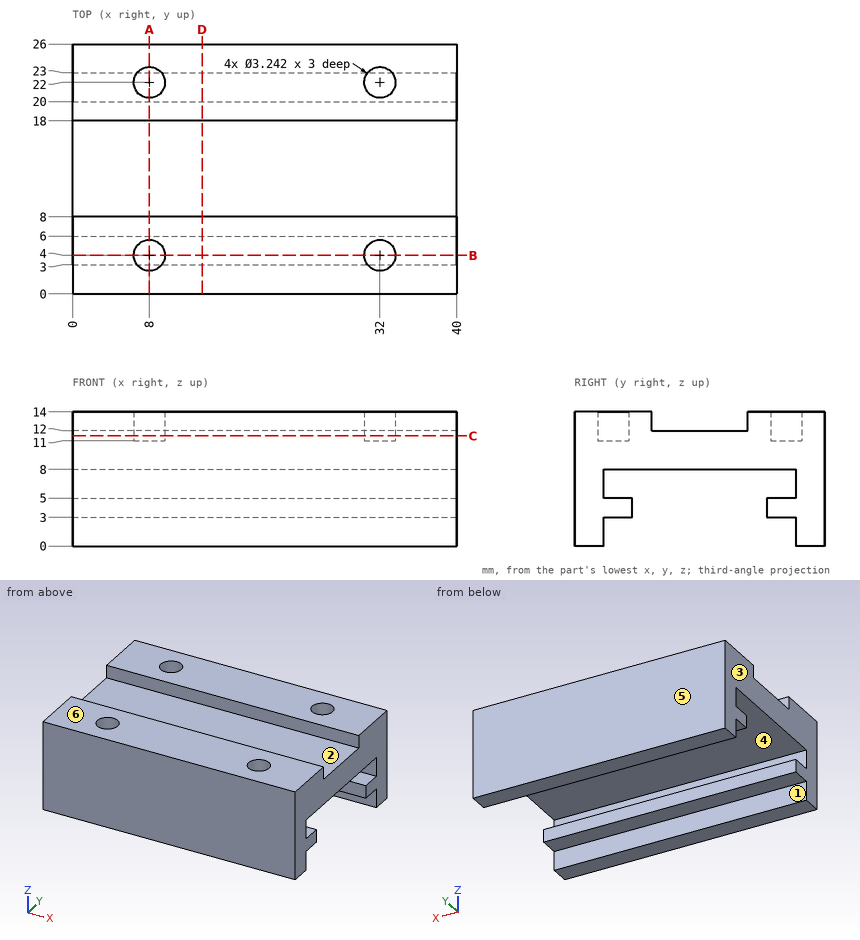
Part print with two shaded views. Sizes in mm from the minimum x, y, z corner. A direction names the side the tool comes from. Coordinates: 2 decimals unless noted, no trailing zeros. Write each loop counter-clockwise with the first axis right and the second up, starting at its lowest first coordinate (ties: lowest second). Pieces come first, ordered by that corner, then holes. Notation, with made-up numbers: (30, 26) - (62, 26) arc R19 cw to (62, 44) - close; hole circle Ø3 at (41.5, -15.75). An arc over 180 degrees is marked (long way). One line per item, written item: value. Start each with the question number.
1. Mould opens along Y. For the marked faces 4, 5 and 6 say: released by +Y, released by -Y, zero draft, split by the parting line, or undercut.
2. Tool access for the marked faces 1, 2 and 3: list every direction of +Z, -Z, +X, -X, +Y, -Y with a clear straight run to the whole face (end or side of a thin tool).
3. Slice it at B-B (y = 4). Write the cut outline in (x, z), plus the area to 3 significant figures.
4. Flat gauge pins, fed straight in: pin 1 (5 mm diameter, centred on x = 26.5, y = 13.5, fed in from +Z); pin 2 (2.5 mm diameter, centred on x = 25.5, y = 21.5, fed in from -Z); pin 3 (1 mm diameter, centred on x = 32.5, y = 4.5, fed in from +Z). Where does each tip first touch, or does it go through?
5. Slice it at C-C (z = 11.5). Write the cut outline in (x, y).
6. Slice it at A-A (x = 8). Write the cut outline in (y, z), plus the area to 3 significant figures.
7. Probe line 1 (Y direction, x = 8, z = 13.35); line 2 (X direction, y = 4, z = 12.95); line 3 (Y direction, x = 32, z = 11.8). List the from-to ranges inside material, lowest first. Write a range as from..to.
8. Slice it at D-D (x = 13.5). Write the cut outline in (y, z).
Answers below:
1. face 4: undercut
1. face 5: released by +Y
1. face 6: zero draft
2. face 1: -Z, +X, -X
2. face 2: +Z, +X, -X
2. face 3: +Z, -Z, -X, +Y, -Y
3. outline: (0, 3) - (40, 3) - (40, 5) - (0, 5) - close; (0, 8) - (40, 8) - (40, 14) - (33.62, 14) - (33.62, 11) - (30.38, 11) - (30.38, 14) - (9.62, 14) - (9.62, 11) - (6.38, 11) - (6.38, 14) - (0, 14) - close
3. area: 301 mm^2
4. pin 1: stops at z = 12
4. pin 2: stops at z = 3
4. pin 3: stops at z = 11
5. outline: (0, 0) - (40, 0) - (40, 26) - (0, 26) - close; hole circle Ø3.24 at (8, 4); hole circle Ø3.24 at (8, 22); hole circle Ø3.24 at (32, 4); hole circle Ø3.24 at (32, 22)
6. outline: (0, 0) - (3, 0) - (3, 3) - (6, 3) - (6, 5) - (3, 5) - (3, 8) - (23, 8) - (23, 5) - (20, 5) - (20, 3) - (23, 3) - (23, 0) - (26, 0) - (26, 14) - (23.62, 14) - (23.62, 11) - (20.38, 11) - (20.38, 14) - (18, 14) - (18, 12) - (8, 12) - (8, 14) - (5.62, 14) - (5.62, 11) - (2.38, 11) - (2.38, 14) - (0, 14) - close
6. area: 177 mm^2
7. line 1: y = 0..2.38, 5.62..8, 18..20.38, 23.62..26
7. line 2: x = 0..6.38, 9.62..30.38, 33.62..40
7. line 3: y = 0..2.38, 5.62..20.38, 23.62..26
8. outline: (0, 0) - (3, 0) - (3, 3) - (6, 3) - (6, 5) - (3, 5) - (3, 8) - (23, 8) - (23, 5) - (20, 5) - (20, 3) - (23, 3) - (23, 0) - (26, 0) - (26, 14) - (18, 14) - (18, 12) - (8, 12) - (8, 14) - (0, 14) - close
